Check sheet for the modelled part. Datum: model origin and axes. Units: mm. Face numbers are marked on the shaded views. A direction names the side the tool comes from. Round coordinates to 2 decimals unless told otherwise and drop trailing zeros. Loops run counter-clockwise (first coordinate to the right, second up) from the corner with the lowest first, then second, coordinate; pieces in that order, holes last. Notation, with made-up numbers: (87.25, 31.5) - (107.25, 31.5) arc R11 cw to (107.25, 52.5) - close; hole circle Ø2 at (-23.75, 33.5). An arc over 180 degrees is marked (long way). Put each result on its own line as item: value. Start each with the question number.
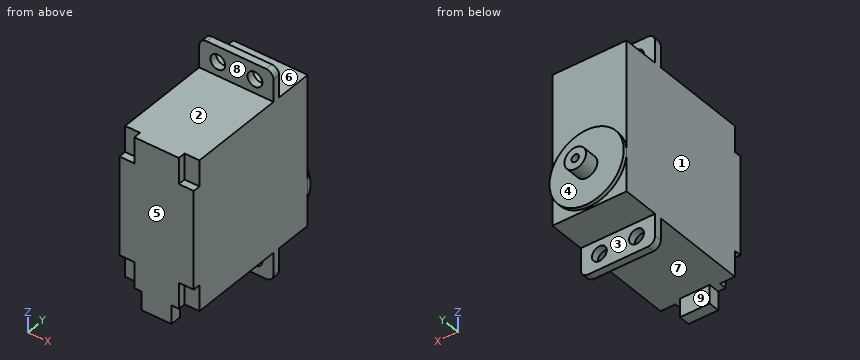
```python
from build123d import *

# Parameters (mm, degrees)
SKETCH2_W           = 20
SKETCH2_H           = 40.5
BOSS_EXTRUDE1_DEPTH = 28
SKETCH3_W           = 20
SKETCH3_H           = 56.4
BOSS_EXTRUDE2_DEPTH = 2
SKETCH4_W           = 20
SKETCH4_H           = 40.5
BOSS_EXTRUDE3_DEPTH = 10
SKETCH5_R           = 10
BOSS_EXTRUDE4_DEPTH = 1
SKETCH6_R           = 2.9
SKETCH6_R_2         = 1
BOSS_EXTRUDE5_DEPTH = 4
SKETCH7_R           = 2
CUT_EXTRUDE1_DEPTH  = 2
FILLET1_R           = 2
SKETCH8_W           = 4
SKETCH8_H           = 7
CUT_EXTRUDE2_DEPTH  = 2
SKETCH9_W           = 8
SKETCH9_H           = 3
BOSS_EXTRUDE6_DEPTH = 5


with BuildPart() as part:
    # Sketch2 → Boss-Extrude1 (new body)
    with BuildSketch(Plane(origin=(0, 77, 0), x_dir=(1, 0, 0), z_dir=(0, 1, 0))):
        with Locations((-39.282617367, 276.14521975)):
            Rectangle(SKETCH2_W, SKETCH2_H)
    extrude(amount=BOSS_EXTRUDE1_DEPTH)

    # Sketch3 → Boss-Extrude2 (add)
    with BuildSketch(Plane(origin=(0, 105, 0), x_dir=(1, 0, 0), z_dir=(0, 1, 0))):
        with Locations((-39.282617367, 276.14521975)):
            Rectangle(SKETCH3_W, SKETCH3_H)
    extrude(amount=BOSS_EXTRUDE2_DEPTH)

    # Sketch4 → Boss-Extrude3 (add)
    with BuildSketch(Plane(origin=(0, 107, 0), x_dir=(1, 0, 0), z_dir=(0, 1, 0))):
        with Locations((-39.282617367, 276.14521975)):
            Rectangle(SKETCH4_W, SKETCH4_H)
    extrude(amount=BOSS_EXTRUDE3_DEPTH)

    # Sketch5 → Boss-Extrude4 (add)
    with BuildSketch(Plane(origin=(0, 117, 0), x_dir=(1, 0, 0), z_dir=(0, 1, 0))):
        with Locations((-39.282617367, 285.89521975)):
            Circle(SKETCH5_R)
    extrude(amount=BOSS_EXTRUDE4_DEPTH)

    # Sketch6 → Boss-Extrude5 (add)
    with BuildSketch(Plane(origin=(0, 118, 0), x_dir=(1, 0, 0), z_dir=(0, 1, 0))):
        with Locations((-39.282617367, 285.89521975)):
            Circle(SKETCH6_R)
        with Locations((-39.282617367, 285.89521975)):
            Circle(SKETCH6_R_2, mode=Mode.SUBTRACT)
    extrude(amount=BOSS_EXTRUDE5_DEPTH)

    # Sketch7 → Cut-Extrude1 (cut)
    with BuildSketch(Plane(origin=(0, 107, 0), x_dir=(1, 0, 0), z_dir=(0, 1, 0))):
        with Locations((-44.282617367, 252.14521975)):
            Circle(SKETCH7_R)
        with Locations((-34.282617367, 252.14521975)):
            Circle(SKETCH7_R)
        with Locations((-34.282617367, 300.14521975)):
            Circle(SKETCH7_R)
        with Locations((-44.282617367, 300.14521975)):
            Circle(SKETCH7_R)
    extrude(amount=-CUT_EXTRUDE1_DEPTH, mode=Mode.SUBTRACT)

    # Fillet1
    fillet1_edges = [part.edges().sort_by_distance(p)[0] for p in [
        (-49.282617367, 106, -247.94521975),
        (-29.282617367, 106, -247.94521975),
        (-49.282617367, 106, -304.34521975),
        (-29.282617367, 106, -304.34521975),
    ]]
    fillet(fillet1_edges, radius=FILLET1_R)

    # Sketch8 → Cut-Extrude2 (cut)
    with BuildSketch(Plane.XZ.offset(-77)):
        with Locations((-31.282617367, -259.39521975)):
            Rectangle(SKETCH8_W, SKETCH8_H)
        with Locations((-31.282617367, -292.89521975)):
            Rectangle(SKETCH8_W, SKETCH8_H)
        with Locations((-47.282617367, -292.89521975)):
            Rectangle(SKETCH8_W, SKETCH8_H)
        with Locations((-47.282617367, -259.39521975)):
            Rectangle(SKETCH8_W, SKETCH8_H)
    extrude(amount=-CUT_EXTRUDE2_DEPTH, mode=Mode.SUBTRACT)

    # Sketch9 → Boss-Extrude6 (add)
    with BuildSketch(Plane(origin=(0, 0, -296.39521975), x_dir=(-1, 0, 0), z_dir=(0, 0, -1))):
        with Locations((39.282617367, 78.5)):
            Rectangle(SKETCH9_W, SKETCH9_H)
    extrude(amount=BOSS_EXTRUDE6_DEPTH)


solid = part.part
```
Q1. Draft check along Y on the marked faces 6, 7, 8 and 9. Enter one of: +Y half, -Y half, draft (parallel to the pull), parting line (faces both ways), or undercut.
Q2. Set-up check for the marked faces 1, 2, 3, 4 and 5: record each of +Z, -Z, +X, -X, +Y, -Y from which the full face is reachable in a straight line by a thin tool's end or side.
Q3. Depth check by flat-ended pin: pin 1 Ø2.5 at (x, z) = (-42, -298.5) entering from +Y; pin 2 Ø1.5 at (y, z) = (78.5, -299.5) entering from +X; pin 3 Ø2 at (y, z) = (77.5, -259) entering from +X; pin 4 Ø4.5 at (x, z) = (-47.5, -260) entering from -Y. Enter the tip coordinate at first touch or a pass-through.
Q4. Cross-section at D-D on y = 119.5. Enter the section's corners in (x, z).
Q5. Cross-section at B-B on z = -260.5. Enter the section's corners in (x, y).
Q6. Material ranges on line 1 (Y direction, x = -43, z = -298.5); line 2 (Z direction, x = -35.25, y = 113.5); line 3 (Y direction, x = -41, z = -288.5), recorded low to high. Write a range as from..to.
Q7. Cross-section at C-C on x = -34.5. Enter the section's corners in (y, z).
Q8. Cross-section at A-A on z = -297. Enter the section's corners in (x, y).
Answer list:
1. face 6: draft
1. face 7: undercut
1. face 8: -Y half
1. face 9: undercut
2. face 1: +Z, -Z, -X, +Y, -Y
2. face 2: +Z, +X, -X, -Y
2. face 3: -Z, +X, -X, +Y
2. face 4: +Y
2. face 5: +Z, -Z, +X, -X, -Y
3. pin 1: stops at y = 107
3. pin 2: stops at x = -35.28
3. pin 3: stops at x = -33.28
3. pin 4: stops at y = 77
4. outline: circle Ø5.8 at (-39.28, -285.9); hole circle Ø2 at (-39.28, -285.9)
5. outline: (-49.28, 79) - (-45.28, 79) - (-45.28, 77) - (-33.28, 77) - (-33.28, 79) - (-29.28, 79) - (-29.28, 117) - (-49.28, 117) - close
6. line 1: y = 77..80, 105..107
6. line 2: z = -296.4..-255.9
6. line 3: y = 77..118
7. outline: (77, -296.4) - (105, -296.4) - (105, -298.16) - (107, -298.16) - (107, -296.4) - (117, -296.4) - (117, -294.68) - (118, -294.68) - (118, -277.11) - (117, -277.11) - (117, -255.9) - (107, -255.9) - (107, -254.13) - (105, -254.13) - (105, -255.9) - (77, -255.9) - close; (105, -304.35) - (107, -304.35) - (107, -302.13) - (105, -302.13) - close; (105, -250.16) - (107, -250.16) - (107, -247.95) - (105, -247.95) - close
8. outline: (-49.28, 105) - (-29.28, 105) - (-29.28, 107) - (-49.28, 107) - close; (-43.28, 77) - (-35.28, 77) - (-35.28, 80) - (-43.28, 80) - close
